Autodesk Inventor part; units mm, degrees
ref_plane "YZ Plane" through (0, 0, 0) normal (1, 0, 0) x (0, 1, 0)
ref_plane "XZ Plane" through (0, 0, 0) normal (0, 1, 0) x (-1, 0, 0)
ref_plane "XY Plane" through (0, 0, 0) normal (0, 0, 1) x (1, 0, 0)
sketch "Sketch1" plane through (0, 0, 0) normal (0, 0, 1) x (1, 0, 0)
  circle A0 centre (0, 0) radius 111.125
  dimension "d0" = 222.25
extrude "Extrusion1" add sketch "Sketch1" along normal blind 12.7
sketch "Sketch2" plane through (0, 0, 12.7) normal (0, 0, 1) x (1, 0, 0)
  circle A0 centre (0, 0) radius 111.125
  circle A1 centre (0, 0) radius 88.9
  circle A2 centre (0, 0) radius 12.7
  dimension "d3" = 177.8
  dimension "d4" = 25.4
extrude "Extrusion2" cut sketch "Sketch2" against normal blind 7.9375 contours A1
sketch "Sketch3" plane through (0, 0, 12.7) normal (0, 0, 1) x (1, 0, 0)
  circle A0 centre (0, 0) radius 12.7
hole "Hole1" at (0, 0, 12.7) direction (0, 0, -1) diameter 12.7 end through all
sketch "Sketch4" plane through (0, 0, 4.7625) normal (0, 0, 1) x (1, 0, 0)
  circle A0 centre (0, 0) radius 12.7
  line L0 (73.025, 3.175) -> (79.375, 3.175)
  line L1 (79.375, 3.175) -> (79.375, -3.175)
  line L2 (79.375, -3.175) -> (73.025, -3.175)
  line L3 (73.025, -3.175) -> (73.025, 3.175)
  circle A1 centre (76.2, 0) radius 3.175 construction
  circle A2 centre (0, 0) radius 6.35
  dimension "d14" = 76.2
  dimension "d15" = 6.35
extrude "Extrusion3" add sketch "Sketch4" along normal blind 6.6675 contours L0 L1 L2 L3
sketch "Sketch5" plane through (0, 0, 0) normal (0, 0, -1) x (-1, 0, 0)
  circle A0 centre (0, 0) radius 6.35
  circle A1 centre (0, 0) radius 111.125
  circle A2 centre (0, 0) radius 9.525
  dimension "d18" = 19.05
extrude "Extrusion4" cut sketch "Sketch5" against normal blind 3.81 contours A2
properties part number "base"
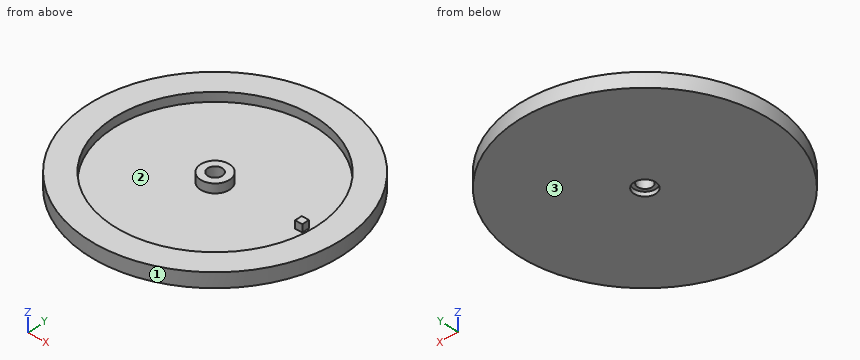
Work out the finished part from the listing and answer in its coordinate system (mm). Face numbers are marked on the shaded views. Give positions to 0.01 mm unless a question says otherwise; leave off trailing zeros. Write each loop counter-clockwise with the first axis right and the second up, starting at its lowest first coordinate (ties: lowest second). Pieces come first, ordered by that corner, then holes.
Q1. Straight lines are drawn through the part: L1, parallel to Y at x = 0, z = 7 (3 decimals); L2, parallel to Y at x = 0, z = 3.05 (3 decimals); L3, parallel to Z at x = 71.5, y = 28. For each, find the intervals that lie inside material, in ascending order.
Answer:
L1: y = -111.125 to -88.9, -12.7 to -6.35, 6.35 to 12.7, 88.9 to 111.125
L2: y = -111.125 to -9.525, 9.525 to 111.125
L3: z = 0 to 4.76
Q2. For a pull along Y with two mould halves and no side action, classify the marked faces 1, 2 and 3 as released by +Y, released by -Y, zero draft, split by the parting line, or undercut.
Answer:
face 1: split by the parting line
face 2: undercut
face 3: zero draft
Q3. The part is cut by section D-D on y = 43.5. Give the vertices of the cut face in (x, z), and give its area (3 significant figures).
Answer:
outline: (-102.26, 0) - (102.26, 0) - (102.26, 12.7) - (77.53, 12.7) - (77.53, 4.76) - (-77.53, 4.76) - (-77.53, 12.7) - (-102.26, 12.7) - close
area: 1,370 mm2
Q4. Given pin 1 (1.5 mm diameter, centred on x = -15.5, z = 4.5, fed in from +Y); pin 2 (7 mm diameter, centred on x = 76.5, z = 8.5, fed in from +Y); pin 3 (1 mm diameter, centred on x = -9, z = 2.5, fed in from +Y); pin 4 (9.5 mm diameter, centred on x = 0, y = 1, fed in from -Z), each flat-ended and moving along its own axis, determine where each tip first touches the part or whether it passes through.
Answer:
pin 1: stops at y = 110.14
pin 2: stops at y = 83.78
pin 3: stops at y = 110.8
pin 4: passes through
Q5. The part is cut by section A-A on z = 9.25. Give the vertices of the cut face in (x, y) (3 decimals).
Answer:
outline: circle Ø222.25 at (0, 0); circle Ø25.4 at (0, 0); (73.025, -3.175) - (79.375, -3.175) - (79.375, 3.175) - (73.025, 3.175) - close; hole circle Ø177.8 at (0, 0); hole circle Ø12.7 at (0, 0)
